Here's the drawing with two shaded views (mm, measured from the low corner). I have some questions. A direction names the side the tool comes from. Give positions to 0.01 mm unless a question says otherwise; leave off trailing zeros. Loops run counter-clockwise (first coordinate to the right, second up) from the corner with the lowest first, then second, coordinate; pieces in that order, holes last.
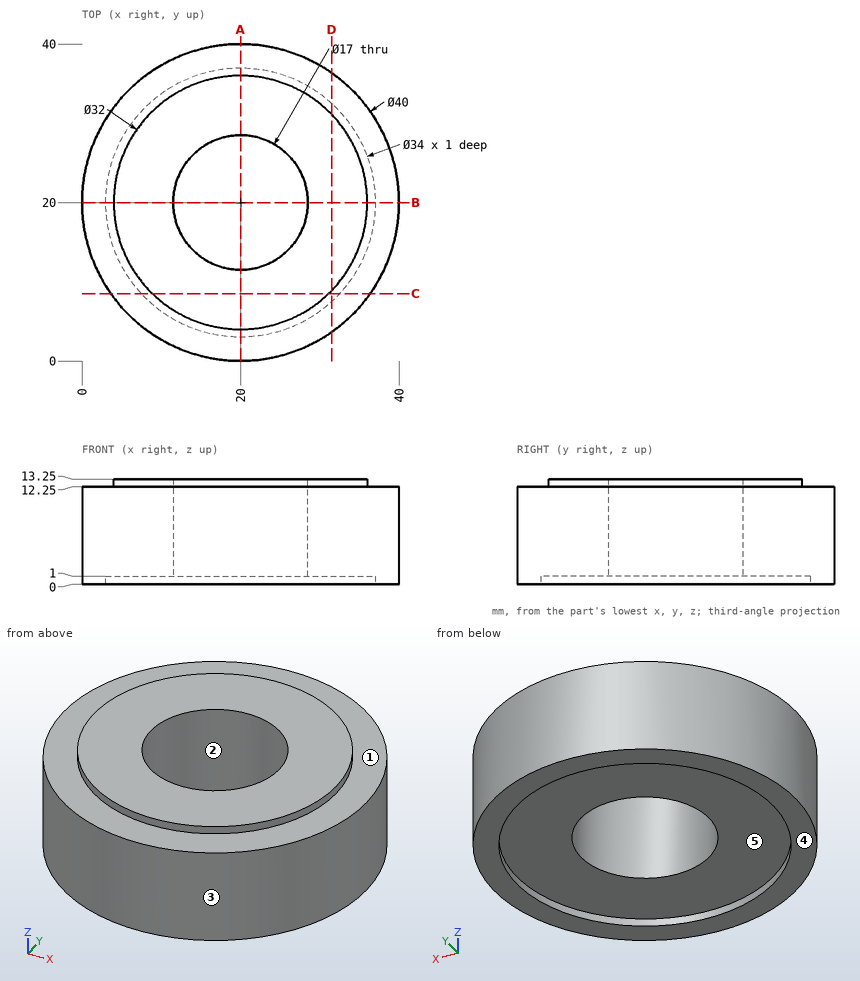
(1) Which directions (+Z, -Z, +X, -X, +Y, -Y) give clear straight access to the entire face, cutting with the end or side of a thin tool? Please do the marked faces 1 and 2.
Returned:
face 1: +Z
face 2: +Z, -Z
(2) Suppose I cut it at A-A on x = 20. List the corners of the cut face in (y, z) for me.
Returned:
outline: (0, 0) - (3, 0) - (3, 1) - (11.5, 1) - (11.5, 13.25) - (4, 13.25) - (4, 12.25) - (0, 12.25) - close; (28.5, 1) - (37, 1) - (37, 0) - (40, 0) - (40, 12.25) - (36, 12.25) - (36, 13.25) - (28.5, 13.25) - close
(3) Suppose I cut it at C-C on y = 8.5. List the corners of the cut face in (x, z) for me, plus the area to 3 significant figures.
Returned:
outline: (3.64, 0) - (7.48, 0) - (7.48, 1) - (32.52, 1) - (32.52, 0) - (36.36, 0) - (36.36, 12.25) - (31.12, 12.25) - (31.12, 13.25) - (8.88, 13.25) - (8.88, 12.25) - (3.64, 12.25) - close
area: 398 mm2
(4) Will these pins go through, and if not, where does the flat tip stop? P1, Ø1.5, axis at y = 33.5, z = 2, coming from the +X side; P2, Ø2, axis at y = 4.5, z = 9.5, coming from the +X side (3 decimals); P3, Ø2, axis at y = 10.5, z = 2.5, coming from the -X side.
Returned:
P1: stops at x = 35.41
P2: stops at x = 33.775
P3: stops at x = 1.9
(5) Thinking about a two-plate mould opening in X: for the marked faces 3, 4 and 5, which applies, pulls with the +X half, pulls with the -X half, needs draft (parallel to the pull), parting line crosses it, or undercut?
Returned:
face 3: parting line crosses it
face 4: needs draft
face 5: undercut
(6) Please list where these lines run through material, in increasing order: probe 1 along Y at (x, z) = (20, 4.75); probe 2 along Y at (x, z) = (20, 0.65).
Returned:
probe 1: y = 0 to 11.5, 28.5 to 40
probe 2: y = 0 to 3, 37 to 40
